```python
from build123d import *

# Parameters (mm, degrees)
PAD_DEPTH = 3


with BuildPart() as part:
    # Sketch → Pad (new body)
    with BuildSketch(Plane.XY):
        with BuildLine():
            ThreePointArc((-2, -0.138593), (-10.937318, -4.980279), (-14.5, -14.499988))
            Line((-14.5, -14.499988), (-14.5, -29.5))
            ThreePointArc((-14.5, -29.5), (6e-06, -44), (14.5, -29.499988))
            Line((14.5, -14.499962), (14.5, -29.499988))
            ThreePointArc((14.5, -14.499962), (10.937309, -4.980269), (2, -0.138593))
            Line((2, -0.138593), (2, 1.861407))
            Line((2, 1.861407), (-2, 1.861407))
            Line((-2, 1.861407), (-2, -0.138593))
        make_face()
        with BuildLine():
            ThreePointArc((13.75, -14.499989), (0, -0.75), (-13.75, -14.499989))
            Line((-13.75, -14.499989), (-13.75, -29.500003))
            ThreePointArc((-13.75, -29.500003), (1e-06, -43.25), (13.75, -29.5))
            Line((13.75, -14.499989), (13.75, -29.5))
        make_face(mode=Mode.SUBTRACT)
    extrude(amount=PAD_DEPTH)


solid = part.part
```
The model under review builds one solid part; all positions refer to its coordinate system, in mm. A direction names the side the tool comes from. Round coordinates to 2 decimals unless told otherwise and drop trailing zeros. Order: outer loops, then holes, each group sorted by start corner. A loop starts at its lowest first (then second) coordinate and runs counter-clockwise, first axis right, second up.
(1) Wall thickness on L1, parallel to X at y = -18, z = 1.5; L2, parallel to X at y = -42, z = 0.3; L3, parallel to Y at x = 8, z = 0.5: over which ranges is each line inside the solid? List them lowest first.
Working result:
L1: x = -14.5 to -13.75, 13.75 to 14.5
L2: x = -7.35 to -5.73, 5.73 to 7.35
L3: y = -41.59 to -40.68, -3.32 to -2.41
(2) Take a section at A-A, the plane y = -18. State the section outline as (x, z) points, plus the area to 3 significant figures.
Working result:
outline: (-14.5, 0) - (-13.75, 0) - (-13.75, 3) - (-14.5, 3) - close; (13.75, 0) - (14.5, 0) - (14.5, 3) - (13.75, 3) - close
area: 4.50 mm2
(3) Mouldability with a two-part tool opening along X and no side actions: class faces 1 (the face through (-10.84, -4.87, 1.48)), 2 (the face through (13.75, -22, 1)), 3 (the face through (14.5, -22, 1)), 4 (the face through (0, 1.861, 1)) as released by +X, released by -X, zero draft, split by the parting line, or undercut.
Working result:
face 1: released by -X
face 2: undercut
face 3: released by +X
face 4: zero draft
(4) Take a section at B-B, the plane z = 0.8. State the section outline as (x, y) points.
Working result:
outline: (-14.5, -29.5) arc R14.5 ccw to (14.5, -29.5) - (14.5, -14.5) arc R14.5 ccw to (2, -0.14) - (2, 1.86) - (-2, 1.86) - (-2, -0.14) arc R14.5 ccw to (-14.5, -14.5) - close; hole (-13.75, -29.5) arc R13.75 ccw to (13.75, -29.5) - (13.75, -14.5) arc R13.75 ccw to (-13.75, -14.5) - close
(5) Take a section at C-C, the plane x = -2.75. State the section outline as (y, z) points.
Working result:
outline: (-43.74, 0) - (-42.97, 0) - (-42.97, 3) - (-43.74, 3) - close; (-1.03, 0) - (-0.26, 0) - (-0.26, 3) - (-1.03, 3) - close
(6) Tool access review of faces 5 (the face through (2, 1, 1)), 6 (the face through (-2, 1, 1)), 7 (the face through (-13.75, -22, 1)), 8 (the face through (14, -19, 0)): name each direction out of +Z, -Z, +X, -X, +Y, -Y from which nothing blocks a thin tool from reaching the whole face with its end or side.
Working result:
face 5: +Z, -Z, +X, +Y
face 6: +Z, -Z, -X, +Y
face 7: +Z, -Z
face 8: -Z, +X, -X, +Y, -Y
(7) For P1, Ø1, axis at y = 1, z = 1.5, coming from the -X side; P2, Ø0.6, axis at y = 1.5, z = 1.5, coming from the +X side, all flat-tipped, find the tip position at first contact; note any pin that passes through.
Working result:
P1: stops at x = -2
P2: stops at x = 2
